Verification items for the finished model (mm, model axes). Face numbers are marked on the shaded views. A direction names the side the tool comes from. Give positions to 0.01 mm unless a question says otherwise; leave off trailing zeros. Order: outer loops, then holes, each group sorted by start corner. A loop starts at its lowest first (then second) coordinate and runs counter-clockwise, first axis right, second up.
(1) Gauge pin test, flat ends, axial feed: pin 1 (5 mm diameter, centred on x = -17.5, y = 32, fed in from -Z); pin 2 (8 mm diameter, centred on y = 4.5, z = 17.5, fed in from -X); pin 3 (4 mm diameter, centred on x = -39.5, z = 8.5, fed in from +Y); pin 4 (6 mm diameter, centred on x = -42.5, y = 28, fed in from -Z). Record the tip position at first contact, or that the pin passes through.
(2) Mould release check, pull along Z, two halves, no side actions. Record for the marked faces 4, 5 and 6: pulls with the +Z half, pulls with the -Z half, needs draft (parallel to the pull), parting line crosses it, or undercut.
(3) Sectioned sample at A-A on x = -27.1. Record the cut outline in (y, z).
(4) Sectioned sample at C-C on z = 16. Record the cut outline in (x, y), plus the area to 3 significant figures.
(5) Scan lines: L1, parallel to Y at x = -27.1, z = 14.25; L2, parallel to Y at x = -27.1, z = 22.5; L3, parallel to X at y = 16.5, z = 10. Record each from-to range of solid material in increasing order.
(6) Sectioned sample at D-D on y = 35. Record the cut outline in (x, z), plus the area to 3 significant figures.
(7) Access from +Z, -Z, +X, -X, +Y, -Y to the whole of each face (thin tool, end or side, straight path). Record for the marked faces 1, 2 and 3.
(8) Sectioned sample at B-B on z = 27. Record the cut outline in (x, y), plus the area to 3 significant figures.
```python
from build123d import *

# Parameters (mm, degrees)
SKETCH1_W           = 54.2
SKETCH1_H           = 25
BOSS_EXTRUDE1_DEPTH = 25
BOSS_EXTRUDE2_DEPTH = 5
FILLET1_R           = 10
FILLET2_R           = 10
CUT_EXTRUDE1_DEPTH  = 20.5
SKETCH5_R           = 2.75
CUT_EXTRUDE2_DEPTH  = 30


with BuildPart() as part:
    # Sketch1 → Boss-Extrude1 (new body)
    with BuildSketch(Plane.XY):
        with Locations((-27.1, 12.5)):
            Rectangle(SKETCH1_W, SKETCH1_H)
        Polygon((-46.2, 4), (-49.516680193, 22.809828083), (-45.577449181, 23.504420793), (-42.843601475, 8), (-11.356398525, 8), (-8.622550819, 23.504420793), (-4.683319807, 22.809828083), (-8, 4), align=None, mode=Mode.SUBTRACT)
        with BuildLine():
            Line((-54.2, 25), (0, 25))
            Line((0, 25), (0, 40))
            Line((0, 40), (-16.1, 40))
            ThreePointArc((-16.1, 40), (-27.1, 29), (-38.1, 40))
            Line((-38.1, 40), (-54.2, 40))
            Line((-54.2, 40), (-54.2, 25))
        make_face()
    extrude(amount=BOSS_EXTRUDE1_DEPTH)

    # Sketch2 → Boss-Extrude2 (add)
    with BuildSketch(Plane.XY.offset(25)):
        with BuildLine():
            Line((-54.2, 40), (-54.2, 0))
            Line((-54.2, 0), (0, 0))
            Line((0, 0), (0, 40))
            Line((0, 40), (-16.1, 40))
            ThreePointArc((-16.1, 40), (-27.1, 29), (-38.1, 40))
            Line((-38.1, 40), (-54.2, 40))
        make_face()
    extrude(amount=BOSS_EXTRUDE2_DEPTH)

    # Fillet1
    fillet1_edges = [part.edges().sort_by_distance(p)[0] for p in [
        (0, 0, 15),
        (-54.2, 0, 15),
    ]]
    fillet(fillet1_edges, radius=FILLET1_R)

    # Fillet2
    fillet2_edges = [part.edges().sort_by_distance(p)[0] for p in [
        (-54.2, 40, 15),
        (0, 40, 15),
    ]]
    fillet(fillet2_edges, radius=FILLET2_R)

    # Sketch4 → Cut-Extrude1 (cut)
    with BuildSketch(Plane(origin=(0, 0, 0), x_dir=(-1, 0, 0), z_dir=(0, 0, -1))):
        with BuildLine():
            ThreePointArc((38.1, 40), (27.1, 29), (16.1, 40))
            Line((16.1, 40), (0, 40))
            Line((0, 40), (0, 24))
            Line((0, 24), (2, 24))
            ThreePointArc((2, 24), (6.790667282, 27.568390069), (11.581334564, 24))
            Line((11.581334564, 24), (42.618665436, 24))
            ThreePointArc((42.618665436, 24), (47.409332718, 27.568390069), (52.2, 24))
            Line((52.2, 24), (54.2, 24))
            Line((54.2, 24), (54.2, 40))
            Line((54.2, 40), (38.1, 40))
        make_face()
    extrude(amount=-CUT_EXTRUDE1_DEPTH, mode=Mode.SUBTRACT)

    # Sketch5 → Cut-Extrude2 (cut)
    with BuildSketch(Plane(origin=(0, 0, 0), x_dir=(-1, 0, 0), z_dir=(0, 0, -1))):
        with Locations((27.1, 16)):
            Circle(SKETCH5_R)
    extrude(amount=-CUT_EXTRUDE2_DEPTH, mode=Mode.SUBTRACT)


solid = part.part
```
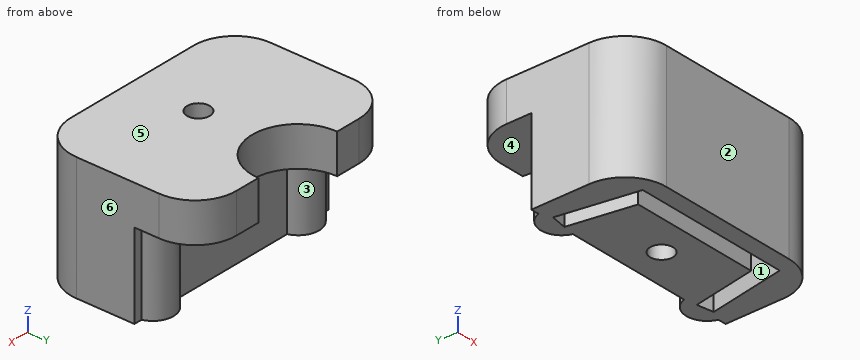
Ans:
1. pin 1: stops at z = 20.5
1. pin 2: stops at x = -54.09
1. pin 3: stops at y = 24
1. pin 4: stops at z = 0
2. face 4: pulls with the -Z half
2. face 5: pulls with the +Z half
2. face 6: needs draft
3. outline: (0, 0) - (4, 0) - (4, 25) - (8, 25) - (8, 0) - (13.25, 0) - (13.25, 30) - (0, 30) - close; (18.75, 0) - (24, 0) - (24, 20.5) - (29, 20.5) - (29, 30) - (18.75, 30) - close
4. outline: (-54.2, 10) arc R10 ccw to (-44.2, 0) - (-10, 0) arc R10 ccw to (0, 10) - (0, 24) - (-2, 24) arc R5 ccw to (-11.58, 24) - (-42.62, 24) arc R5 ccw to (-52.2, 24) - (-54.2, 24) - close; hole (-49.52, 22.81) - (-46.2, 4) - (-8, 4) - (-4.68, 22.81) - (-8.62, 23.5) - (-11.36, 8) - (-42.84, 8) - (-45.58, 23.5) - close; hole circle Ø5.5 at (-27.1, 16)
4. area: 1,010 mm2
5. L1: y = 0 to 4, 8 to 13.25, 18.75 to 24
5. L2: y = 0 to 4, 8 to 13.25, 18.75 to 29
5. L3: x = -54.2 to -48.4, -44.34 to -29.8, -24.4 to -9.86, -5.8 to 0
6. outline: (-52.86, 20.5) - (-36.9, 20.5) - (-36.9, 30) - (-52.86, 30) - close; (-17.3, 20.5) - (-1.34, 20.5) - (-1.34, 30) - (-17.3, 30) - close
6. area: 303 mm2
7. face 1: -Z
7. face 2: +Z, -Z, +X, -X, -Y
7. face 3: -Z, +Y
8. outline: (-54.2, 10) arc R10 ccw to (-44.2, 0) - (-10, 0) arc R10 ccw to (0, 10) - (0, 30) arc R10 ccw to (-10, 40) - (-16.1, 40) arc R11 cw to (-38.1, 40) - (-44.2, 40) arc R10 ccw to (-54.2, 30) - close; hole circle Ø5.5 at (-27.1, 16)
8. area: 1,870 mm2
